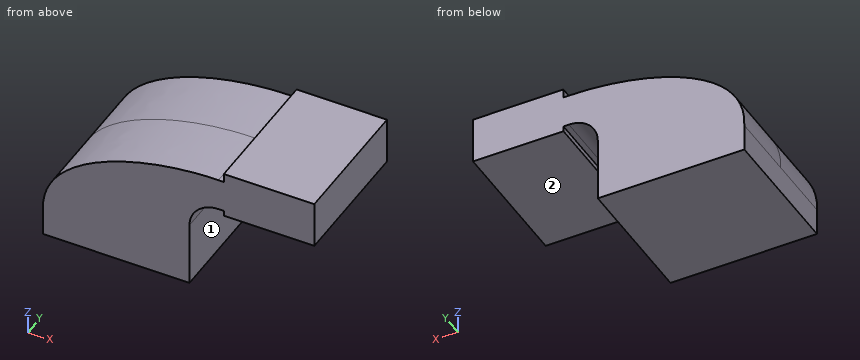
from build123d import *

# Parameters (mm, degrees)
F0_W     = 25
F0_H     = 5
F0_H_2   = 18
F0_H_3   = 3
F1_DEPTH = 37.5


with BuildPart() as f1:
    # F0 (on Front) → F1 (new body, symmetric)
    with BuildSketch(Plane.XZ):
        with BuildLine():
            Line((-40.5, 7.5), (22.5, 7.5))
            Line((22.5, 7.5), (22.5, 28.5))
            ThreePointArc((22.5, 28.5), (32.4583694397, 52.5416305603), (56.5, 62.5))
            add(Edge.make_bspline(
                [(-40.5, 7.5), (-42.4130707979, 45.3152880073), (14.8186171427, 63.0258098245), (56.5, 62.5)],
                knots=[0, 0, 0, 0, 111.5078472575, 111.5078472575, 111.5078472575, 111.5078472575], degree=3))
        make_face()
        with BuildLine():
            Line((22.5, 7.5), (40.5, 7.5))
            Line((40.5, 7.5), (40.5, 28.5))
            ThreePointArc((40.5, 28.5), (45.186291501, 39.813708499), (56.5, 44.5))
            Line((56.5, 44.5), (59.5, 44.5))
            Line((59.5, 44.5), (59.5, 62.5))
            Line((59.5, 62.5), (56.5, 62.5))
            ThreePointArc((56.5, 62.5), (32.4583694397, 52.5416305603), (22.5, 28.5))
            Line((22.5, 28.5), (22.5, 7.5))
        make_face()
        with Locations((72, 65)):
            Rectangle(F0_W, F0_H)
        with Locations((72, 53.5)):
            Rectangle(F0_W, F0_H_2)
        with Locations((72, 43)):
            Rectangle(F0_W, F0_H_3)
        Polygon((84.5, 62.5), (84.5, 44.5), (84.5, 41.5), (109.5, 41.5), (109.5, 67.5), (84.5, 67.5), align=None)
        Polygon((40.5, -7.5), (40.5, 7.5), (22.5, 7.5), (-40.5, 7.5), (-40.5, -7.5), align=None)
    extrude(amount=F1_DEPTH, both=True)


solid = f1.part
Check sheet for the modelled part. Datum: model origin and axes. Units: mm. Face numbers are marked on the shaded views. Round coordinates to 2 decimals unless told otherwise and drop trailing zeros. Loops run counter-clockwise (first coordinate to the right, second up) from the corner with the lowest first, then second, coordinate; pieces in that order, holes last.
1. Sectioned sample at A-A on z = -2. Record the boundary of the cut face in (x, y).
2. Scan lines: probe 1 along X at (y, z) = (33.5, 0); probe 2 along Z at (x, y) = (78.5, -30); probe 3 along Z at (x, y) = (56.5, -28.5). Record each from-to range of solid material in increasing order.
3. Gauge pin test, flat ends, axial feed: pin 1 Ø0.9 at (x, y) = (57.5, -3.5) entering from +Z; pin 2 Ø7.5 at (y, z) = (4.5, 2) entering from -X; pin 3 Ø25 at (x, y) = (92, -7) entering from -Z. Record the tip position at first contact, or that the pin passes through.
4. Mould release check, pull along X, two halves, no side actions. Record for the marked faces 1 and 2: released by +X, released by -X, zero draft, split by the parting line, or undercut.
Recorded:
1. outline: (-40.5, -37.5) - (40.5, -37.5) - (40.5, 37.5) - (-40.5, 37.5) - close
2. probe 1: x = -40.5 to 40.5
2. probe 2: z = 41.5 to 67.5
2. probe 3: z = 44.5 to 62.5
3. pin 1: stops at z = 62.5
3. pin 2: stops at x = -40.5
3. pin 3: stops at z = 41.5
4. face 1: released by +X
4. face 2: zero draft
